Drawing for the job (mm, zero at the part's lowest x, y, z). A direction names the side the tool comes from. Round coordinates to 2 decimals unless told otherwise and drop trailing zeros. Write each loop counter-clockwise with the first axis right and the second up, starting at its lowest first coordinate (ties: lowest second). Pieces come first, ordered by that corner, then holes. Notation, with made-up numbers: M -5.5,-21 L 53.5,-21 A22 ccw 53.5,-14 Z; hole C 53,33.5 d10. An arc over 180 degrees is marked long. Use a Markdown table: item, result. Add a question column.
1) Wall check: probe 1 along Y at (x, z) = (2092, 71); probe 2 along Z at (x, y) = (1111, 148.5); probe 3 along X at (y, z) = (81, 61.5). Give the ranges that are in metal, low to high.
2) Slice it at A-A on z = 64.5. Write the cut outline in (x, y), plus the area to 3 significant figures.
3) Which spindle directions (+Z, -Z, +X, -X, +Y, -Y) get a long thin tool onto all of the face, cutting with end or side? Do the marked faces 1 and 2. Say none if no direction does.
4) Slice it at B-B on y = 153. Write the cut outline in (x, z), plus the area to 4 significant figures.
5) Drop flat-ended pins along their axis: P1, Ø1.5, axis at x = 1666.5, z = 77, coming from the -Y side; P2, Ø1.5, axis at y = 211.5, z = 50, coming from the -X side; P3, Ø4, axis at x = 1883, y = 251.5, coming from the -Z side. Give the stop position or say it passes through.
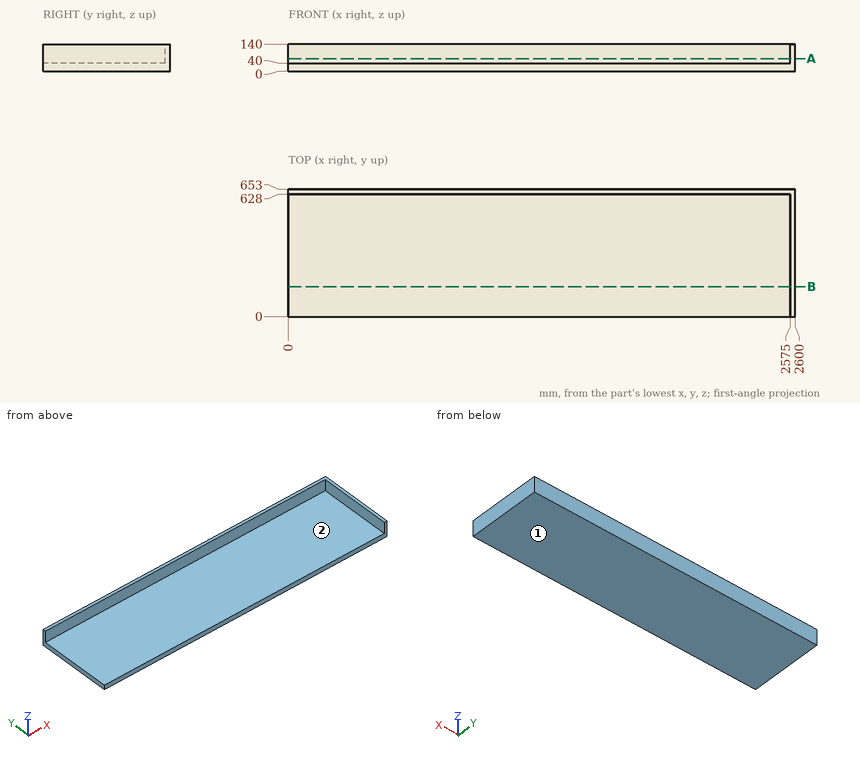
Entries:
| question | item | result |
|---|---|---|
| 1 | probe 1 | y = 628 to 653 |
| 1 | probe 2 | z = 0 to 40 |
| 1 | probe 3 | x = 2575 to 2600 |
| 2 | outline | M 0,628 L 2575,628 L 2575,0 L 2600,0 L 2600,653 L 0,653 Z |
| 2 | area | 80,700 mm^2 |
| 3 | face 1 | -Z, +X, -X, +Y, -Y |
| 3 | face 2 | +Z, -X, -Y |
| 4 | outline | M 0,0 L 2600,0 L 2600,140 L 2575,140 L 2575,40 L 0,40 Z |
| 4 | area | 106,500 mm^2 |
| 5 | P1 | stops at y = 628 |
| 5 | P2 | stops at x = 2575 |
| 5 | P3 | stops at z = 0 |
